from build123d import *

# Parameters (mm, degrees)
F1_DEPTH      = 1.2
F1_DEPTH_BACK = 0.4
F3_DEPTH      = 12.5
F5_DEPTH      = 2
F6_DEPTH      = 5
F7_T2_ANGLE   = 119.2786087223
F8_DEPTH      = 5
F10_DEPTH     = 4
F11_DEPTH     = 5


# Not quite as in the source:
# - a fillet or chamfer that OpenCascade refuses, or shapes differently, is made with other operations: its cross-section is extruded or revolved along the edge and cut away or added
# - a feature names something its author has since deleted; it is built from what else it names


with BuildPart() as f1:
    # F0 (on Top) → F1 (new body, two sides)
    with BuildSketch(Plane.XY) as f1_sk:
        with BuildLine():
            ThreePointArc((-3.25, -2.3318447633), (0, 4), (3.25, -2.3318447633))
            Line((3.25, -2.3318447633), (4.1771243445, -3.8318447633))
            Line((4.1771243445, -3.8318447633), (5.5, -2.3318447633))
            Line((5.5, -2.3318447633), (6.2861850371, 8.4103434936))
            ThreePointArc((6.2861850371, 8.4103434936), (0, 10.5), (-6.2861850371, 8.4103434936))
            Line((-6.2861850371, 8.4103434936), (-5.5, -2.3318447633))
            Line((-5.5, -2.3318447633), (-4.1771243445, -3.8318447633))
            Line((-4.1771243445, -3.8318447633), (-3.25, -2.3318447633))
        make_face()
    extrude(amount=F1_DEPTH)
    extrude(f1_sk.sketch, amount=-F1_DEPTH_BACK)

    # F2 (on Right) → F3 (cut, symmetric)
    with BuildSketch(Plane.YZ):
        Polygon((-3.8318447633, 0.4), (-2.3318447633, 1.2), (-3.8318447633, 1.2), align=None)
    extrude(amount=F3_DEPTH, both=True, mode=Mode.SUBTRACT)

    # F4 (on face) → F5 (join)
    with BuildSketch(Plane.XY.offset(1.2)):
        with BuildLine():
            Line((0, 9.4893432962), (0, 9.5))
            ThreePointArc((0, 9.5), (-1.0056504861, 9.4466219941), (-2, 9.2870878105))
            ThreePointArc((-2, 9.2870878105), (-2.207287093, 9.2400153511), (-2.4134691055, 9.1883168686))
            Line((-2.4134691055, 9.1883168686), (-1.6054997382, 6.2986006851))
            ThreePointArc((-1.6054997382, 6.2986006851), (-0.809041268, 6.4494536378), (0, 6.5))
            Line((0, 6.5), (0, 9.4893432962))
        make_face()
        with BuildLine():
            Line((0, 10.3126084432), (0, 9.5))
            ThreePointArc((0, 9.5), (1.0056504861, 9.4466219941), (2, 9.2870878105))
            Line((2, 9.2870878105), (2, 10.3126084432))
            Line((2, 10.3126084432), (0, 10.3126084432))
        make_face()
        with BuildLine():
            ThreePointArc((2, 9.2870878105), (1.0056504861, 9.4466219941), (0, 9.5))
            Line((0, 9.5), (0, 9.4893432962))
            Line((0, 9.4893432962), (0, 6.5))
            ThreePointArc((0, 6.5), (0.809041268, 6.4494536378), (1.6054997382, 6.2986006851))
            Line((1.6054997382, 6.2986006851), (2.4134691055, 9.1883168686))
            ThreePointArc((2.4134691055, 9.1883168686), (2.207287093, 9.2400153511), (2, 9.2870878105))
        make_face()
        with BuildLine():
            ThreePointArc((-2, 9.2870878105), (-1.0056504861, 9.4466219941), (0, 9.5))
            Line((0, 9.5), (0, 10.3126084432))
            Line((0, 10.3126084432), (-2, 10.3126084432))
            Line((-2, 10.3126084432), (-2, 9.2870878105))
        make_face()
        with BuildLine():
            Line((-1.6054997382, 6.2986006851), (-2.4134691055, 9.1883168686))
            ThreePointArc((-2.4134691055, 9.1883168686), (-4.3834961594, 8.4282240965), (-6.1369591907, 7.2517399217))
            ThreePointArc((-6.1369591907, 7.2517399217), (-6.2072372931, 7.1135226449), (-6.1576144754, 6.9666192642))
            Line((-6.1576144754, 6.9666192642), (-4.3047045796, 4.8702688306))
            Line((-4.3047045796, 4.8702688306), (-4.2185888433, 4.7728389657))
            ThreePointArc((-4.2185888433, 4.7728389657), (-4.0971505607, 4.7073203992), (-3.9621862374, 4.7360357341))
            Line((-3.9621862374, 4.7360357341), (-2.5827247856, 5.6044208159))
            ThreePointArc((-2.5827247856, 5.6044208159), (-2.4942501859, 5.7293355978), (-2.5200172859, 5.8802246764))
            Line((-2.5200172859, 5.8802246764), (-2.5753119947, 5.968062343))
            ThreePointArc((-2.5753119947, 5.968062343), (-2.096928846, 6.152470188), (-1.6054997382, 6.2986006851))
        make_face()
        with BuildLine():
            ThreePointArc((6.1369591907, 7.2517399217), (4.3834961594, 8.4282240965), (2.4134691055, 9.1883168686))
            Line((2.4134691055, 9.1883168686), (1.6054997382, 6.2986006851))
            ThreePointArc((1.6054997382, 6.2986006851), (2.096928846, 6.152470188), (2.5753119947, 5.968062343))
            Line((2.5753119947, 5.968062343), (2.5200172859, 5.8802246764))
            ThreePointArc((2.5200172859, 5.8802246764), (2.4942501859, 5.7293355978), (2.5827247856, 5.6044208159))
            Line((2.5827247856, 5.6044208159), (3.9621862374, 4.7360357341))
            ThreePointArc((3.9621862374, 4.7360357341), (4.0971505607, 4.7073203992), (4.2185888433, 4.7728389657))
            Line((4.2185888433, 4.7728389657), (4.3047045796, 4.8702688306))
            Line((4.3047045796, 4.8702688306), (6.1576144754, 6.9666192642))
            ThreePointArc((6.1576144754, 6.9666192642), (6.2072372931, 7.1135226449), (6.1369591907, 7.2517399217))
        make_face()
    extrude(amount=F5_DEPTH)

    # F4 (on face) → F6 (join)
    with BuildSketch(Plane.XY.offset(1.2)):
        with BuildLine():
            ThreePointArc((2, 9.2870878105), (1.0056504861, 9.4466219941), (0, 9.5))
            Line((0, 9.5), (0, 9.4893432962))
            Line((0, 9.4893432962), (0, 6.5))
            ThreePointArc((0, 6.5), (0.809041268, 6.4494536378), (1.6054997382, 6.2986006851))
            Line((1.6054997382, 6.2986006851), (2.4134691055, 9.1883168686))
            ThreePointArc((2.4134691055, 9.1883168686), (2.207287093, 9.2400153511), (2, 9.2870878105))
        make_face()
        with BuildLine():
            Line((0, 9.4893432962), (0, 9.5))
            ThreePointArc((0, 9.5), (-1.0056504861, 9.4466219941), (-2, 9.2870878105))
            ThreePointArc((-2, 9.2870878105), (-2.207287093, 9.2400153511), (-2.4134691055, 9.1883168686))
            Line((-2.4134691055, 9.1883168686), (-1.6054997382, 6.2986006851))
            ThreePointArc((-1.6054997382, 6.2986006851), (-0.809041268, 6.4494536378), (0, 6.5))
            Line((0, 6.5), (0, 9.4893432962))
        make_face()
    extrude(amount=F6_DEPTH)

    # F7: chamfer of 2 on 1 edges, made by hand

    # F7_s1 → F7_t2 (revolve, cut)
    with BuildSketch(Plane(origin=(0, 0, 0), x_dir=(0, 0, 1), z_dir=(-0.5054419689, -0.8628606006, 0))):
        Polygon((6.2, 8.5), (4.2, 6.5), (6.2, 6.5), align=None)
    revolve(axis=Axis((0, 0, 6.2), (0, 0, -1)), revolution_arc=F7_T2_ANGLE, mode=Mode.SUBTRACT)

    # F4 (on face) → F8 (join, through all)
    with BuildSketch(Plane.XY.offset(1.2)):
        with BuildLine():
            Line((0, 10.3126084432), (0, 9.5))
            ThreePointArc((0, 9.5), (1.0056504861, 9.4466219941), (2, 9.2870878105))
            Line((2, 9.2870878105), (2, 10.307764064))
            ThreePointArc((2, 10.307764064), (1.9874359165, 10.3101939108), (1.974868881, 10.3126084432))
            Line((1.974868881, 10.3126084432), (0, 10.3126084432))
        make_face()
        with BuildLine():
            ThreePointArc((1.974868881, 10.3126084432), (1.9874359165, 10.3101939108), (2, 10.307764064))
            Line((2, 10.307764064), (2, 10.3126084432))
            Line((2, 10.3126084432), (1.974868881, 10.3126084432))
        make_face()
        with BuildLine():
            Line((-2, 10.3126084432), (-2, 10.307764064))
            ThreePointArc((-2, 10.307764064), (-1.9874359165, 10.3101939108), (-1.974868881, 10.3126084432))
            Line((-1.974868881, 10.3126084432), (-2, 10.3126084432))
        make_face()
        with BuildLine():
            ThreePointArc((-2, 9.2870878105), (-1.0056504861, 9.4466219941), (0, 9.5))
            Line((0, 9.5), (0, 10.3126084432))
            Line((0, 10.3126084432), (-1.974868881, 10.3126084432))
            ThreePointArc((-1.974868881, 10.3126084432), (-1.9874359165, 10.3101939108), (-2, 10.307764064))
            Line((-2, 10.307764064), (-2, 9.2870878105))
        make_face()
    extrude(amount=F8_DEPTH)

    # F9 (on face) → F10 (join)
    with BuildSketch(Plane(origin=(-2, 0, 0), x_dir=(0, -1, 0), z_dir=(-1, 0, 0))):
        with BuildLine():
            Line((-10.4906475171, 1.2), (-10.3126084432, 1.2))
            Line((-10.3126084432, 1.2), (-10.3126084432, 6.2))
            ThreePointArc((-10.3126084432, 6.2), (-10.7033019047, 9.142871965), (-11.848315427, 11.8818646297))
            ThreePointArc((-11.848315427, 11.8818646297), (-13.2228522743, 12.2616673302), (-14.6442650052, 12.1468305588))
            ThreePointArc((-14.6442650052, 12.1468305588), (-15.8696799602, 10.6519801079), (-16.5821556002, 8.8551500812))
            ThreePointArc((-16.5821556002, 8.8551500812), (-16.7217466821, 7.8095628414), (-16.5821556002, 6.7639756016))
            ThreePointArc((-16.5821556002, 6.7639756016), (-14.0870903715, 3.3790869985), (-10.4906475171, 1.2))
        make_face()
    extrude(amount=-F10_DEPTH)

    # F4 (on face) → F11 (join, through all)
    with BuildSketch(Plane.XY.offset(1.2)):
        with BuildLine():
            Line((0, 10.3126084432), (0, 9.5))
            ThreePointArc((0, 9.5), (1.0056504861, 9.4466219941), (2, 9.2870878105))
            Line((2, 9.2870878105), (2, 10.307764064))
            ThreePointArc((2, 10.307764064), (1.9874359165, 10.3101939108), (1.974868881, 10.3126084432))
            Line((1.974868881, 10.3126084432), (0, 10.3126084432))
        make_face()
        with BuildLine():
            ThreePointArc((-2, 9.2870878105), (-1.0056504861, 9.4466219941), (0, 9.5))
            Line((0, 9.5), (0, 10.3126084432))
            Line((0, 10.3126084432), (-1.974868881, 10.3126084432))
            ThreePointArc((-1.974868881, 10.3126084432), (-1.9874359165, 10.3101939108), (-2, 10.307764064))
            Line((-2, 10.307764064), (-2, 9.2870878105))
        make_face()
    extrude(amount=F11_DEPTH)


solid = f1.part
Geometry: final body of the model. Coordinates: model frame, mm. A direction names the side the tool comes from. Give positions to 0.01 mm unless a question says otherwise; leave off trailing zeros. Order: outer loops, then holes, each group sorted by start corner. A loop starts at its lowest first (then second) coordinate and runs counter-clockwise, first axis right, second up. Notation, with made-up numbers: (31.25, 63) -> (79.25, 63) arc R26 ccw to (79.25, 90) -> close; hole circle Ø2 at (-7.5, 46.5). An arc over 180 degrees is marked (long way). Answer as a JSON object with one key per item and string values.
Q1. Section B-B (z = 4.5). Output: boundary loops of the cut face in (x, y), plus the area to 3 significant figures.
Entries:
{"outline": "(-2.41, 9.19) -> (-1.69, 6.59) arc R6.8 cw to (1.69, 6.59) -> (2.41, 9.19) arc R9.5 ccw to (2, 9.29) -> (2, 15.15) -> (-2, 15.15) -> (-2, 9.29) arc R9.5 ccw to start", "area": "34.1 mm^2"}
Q2. Section A-A (y = 3.5). Output: boundary loops of the cut face in (x, z), plus the area to 3 significant figures.
Entries:
{"outline": "(-5.93, -0.4) -> (-1.94, -0.4) -> (-1.94, 1.2) -> (-5.93, 1.2) -> close; (1.94, -0.4) -> (5.93, -0.4) -> (5.93, 1.2) -> (1.94, 1.2) -> close", "area": "12.8 mm^2"}
Q3. Section C-C (x = -5). Output: boundary loops of the cut face in (y, z), plus the area to 3 significant figures.
Entries:
{"outline": "(-2.9, -0.4) -> (9.23, -0.4) -> (9.23, 1.2) -> (8.08, 1.2) -> (8.08, 3.2) -> (5.66, 3.2) -> (5.66, 1.2) -> (-2.33, 1.2) -> (-2.9, 0.9) -> close", "area": "24.2 mm^2"}
Q4. Access query for faces 1 (the flat face through (0, 9, 6.2)), 2 (the flat face through (4, 7, 3.2)), 3 (the flat face through (-3.282, 5.164, 2.186)). Directions: +Z, -Z, +X, -X, +Y, -Y. A direction counts if a zero-diameter tool reaches every point of the face in a straight line with its end or side. Return the directions, or none.
Entries:
{"face 1": "+Z, +X, -X, -Y", "face 2": "+Z, +X, -Y", "face 3": "+Z, -Y"}
Q5. First-contact query: pin 1 (1 mm diameter, centred on x = 0.5, y = 9, fed in from +Z); pin 2 (2.5 mm diameter, centred on x = -4, y = 9, fed in from +Z); pin 3 (1 mm diameter, centred on x = -4, y = -1.5, fed in from +Z). Flat tips, straight axial feed; report the tip coordinate or a pass-through.
Entries:
{"pin 1": "stops at z = 6.2", "pin 2": "stops at z = 3.2", "pin 3": "stops at z = 1.2"}
Q6. Material intervals for probe 1 along Y at (x, z) = (0, 0.1); probe 2 along Z at (x, y) = (-4.5, 8.5); probe 3 along X at (y, z) = (0, 0.9), sorted ascending.
Entries:
{"probe 1": "y = 4 to 10.5", "probe 2": "z = -0.4 to 1.2", "probe 3": "x = -5.67 to -4, 4 to 5.67"}
Q7. Section D-D (y = 1). Output: boundary loops of the cut face in (x, z), plus the area to 3 significant figures.
Entries:
{"outline": "(-5.74, -0.4) -> (-3.87, -0.4) -> (-3.87, 1.2) -> (-5.74, 1.2) -> close; (3.87, -0.4) -> (5.74, -0.4) -> (5.74, 1.2) -> (3.87, 1.2) -> close", "area": "5.99 mm^2"}
